The model under review builds one solid part; all positions refer to its coordinate system, in mm. Face numbers are marked on the shaded views. A direction names the side the tool comes from. Coordinates: 2 decimals unless noted, no trailing zeros. Write each loop counter-clockwise with the first axis right and the second up, starting at its lowest first coordinate (ties: lowest second). Pieces come first, ordered by that corner, then holes. Notation, with made-up numbers: (-8, -38.75) -> (14, -38.75) arc R31 ccw to (14, -6.75) -> close; hole circle Ø7 at (16.25, 70). An arc over 180 degrees is marked (long way). Put each result on its own line as item: value. Start each with the question number.
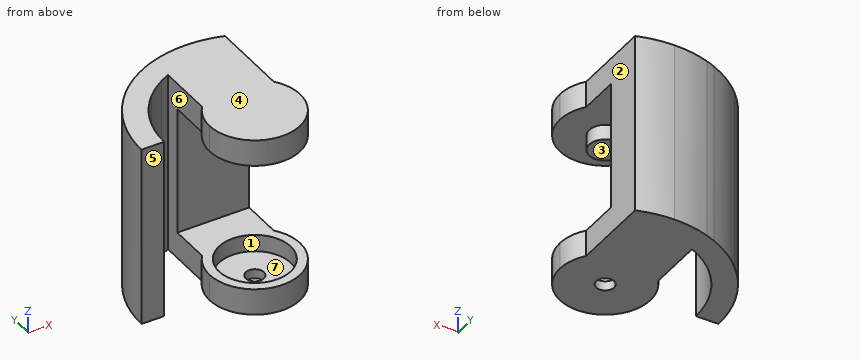
from build123d import *
from build123d.topology import SkipClean

# Parameters (mm, degrees)
SKETCH1_R           = 9.5
BOSS_EXTRUDE1_DEPTH = 48
SKETCH2_W           = 34
SKETCH2_H           = 30
CUT_EXTRUDE1_DEPTH  = 62.481704596
BOSS_EXTRUDE2_START = -2.5
SKETCH3_R           = 9.5
SKETCH3_R_2         = 2.4
BOSS_EXTRUDE2_DEPTH = 2.5
SKETCH4_R           = 9.5
SKETCH4_R_2         = 4.2
BOSS_EXTRUDE3_DEPTH = 7
SKETCH5_R           = 4.2
BOSS_EXTRUDE4_DEPTH = 11
CUT_EXTRUDE2_DEPTH  = 58.861904566
BOSS_EXTRUDE5_DEPTH = 48


with BuildPart() as part:
    # Sketch1 → Boss-Extrude1 (new body)
    with BuildSketch(Plane.XY):
        with BuildLine():
            Line((-12, 0), (-12, 30))
            Line((-12, 30), (12, 30))
            Line((12, 30), (12, 0))
            ThreePointArc((12, 0), (0, -12), (-12, 0))
        make_face()
        Circle(SKETCH1_R, mode=Mode.SUBTRACT)
    extrude(amount=-BOSS_EXTRUDE1_DEPTH)

    # Sketch2 → Cut-Extrude1 (cut, through all)
    with BuildSketch(Plane.ZY.offset(12)):
        with Locations((-24, 3)):
            Rectangle(SKETCH2_W, SKETCH2_H)
    extrude(amount=-CUT_EXTRUDE1_DEPTH, mode=Mode.SUBTRACT)

    # Sketch3 → Boss-Extrude2 (add)
    with BuildSketch(Plane(origin=(0, 0, -48), x_dir=(-1, 0, 0), z_dir=(0, 0, -1)).offset(BOSS_EXTRUDE2_START)):
        Circle(SKETCH3_R)
        Circle(SKETCH3_R_2, mode=Mode.SUBTRACT)
    extrude(amount=BOSS_EXTRUDE2_DEPTH)

    # Sketch4 → Boss-Extrude3 (add)
    with BuildSketch(Plane.XY):
        with Locations(Location((0, 0, 0), (0, 0, 180))):
            Circle(SKETCH4_R)
        Circle(SKETCH4_R_2, mode=Mode.SUBTRACT)
    extrude(amount=-BOSS_EXTRUDE3_DEPTH)

    # Sketch5 → Boss-Extrude4 (add)
    with BuildSketch(Plane.XY):
        Circle(SKETCH5_R)
    extrude(amount=-BOSS_EXTRUDE4_DEPTH)

    # Sketch6 → Cut-Extrude2 (cut, through all)
    with SkipClean():  # the faces are left unmerged after this step: merging them gives an invalid solid
        with BuildSketch(Plane(origin=(0, 0, -48), x_dir=(-1, 0, 0), z_dir=(0, 0, -1))):
            with BuildLine():
                Line((-12, 30), (-12, 27.49545417))
                ThreePointArc((-12, 27.49545417), (-10.760725498, 28.003692377), (-9.5, 28.45610655))
                Line((-9.5, 28.45610655), (-9.5, 30))
                Line((-9.5, 30), (-12, 30))
            make_face()
            with BuildLine():
                Line((-9.5, 30), (-9.5, 28.45610655))
                ThreePointArc((-9.5, 28.45610655), (-4.812317696, 29.611511248), (2.9e-08, 30))
                Line((2.9e-08, 30), (-9.5, 30))
            make_face()
            with BuildLine():
                ThreePointArc((2.9e-08, 30), (4.812317725, 29.611511243), (9.5, 28.45610655))
                Line((9.5, 28.45610655), (9.5, 30))
                Line((9.5, 30), (2.9e-08, 30))
            make_face()
            with BuildLine():
                Line((9.5, 30), (9.5, 28.45610655))
                ThreePointArc((9.5, 28.45610655), (10.760725498, 28.003692377), (12, 27.49545417))
                Line((12, 27.49545417), (12, 30))
                Line((12, 30), (9.5, 30))
            make_face()
            with BuildLine():
                Line((-12, 20.784609691), (-12, 0))
                ThreePointArc((-12, 0), (-11.357816692, 3.872983346), (-9.5, 7.331439149))
                Line((-9.5, 7.331439149), (-9.5, 22.039736841))
                ThreePointArc((-9.5, 22.039736841), (-10.768302375, 21.448628487), (-12, 20.784609691))
            make_face()
            with BuildLine():
                Line((-12, 27.49545417), (-12, 20.784609691))
                ThreePointArc((-12, 20.784609691), (-10.768302375, 21.448628487), (-9.5, 22.039736841))
                Line((-9.5, 22.039736841), (-9.5, 28.45610655))
                ThreePointArc((-9.5, 28.45610655), (-10.760725498, 28.003692377), (-12, 27.49545417))
            make_face()
            with BuildLine():
                Line((9.5, 22.039736841), (9.5, 9.5))
                Line((9.5, 9.5), (12, 12))
                Line((12, 12), (12, 20.784609691))
                ThreePointArc((12, 20.784609691), (10.768302375, 21.448628487), (9.5, 22.039736841))
            make_face()
            with BuildLine():
                ThreePointArc((9.5, 7.331439149), (11.357816692, 3.872983346), (12, 0))
                Line((12, 0), (12, 12))
                Line((12, 12), (9.5, 9.5))
                Line((9.5, 9.5), (9.5, 7.331439149))
            make_face()
        extrude(amount=-CUT_EXTRUDE2_DEPTH, mode=Mode.SUBTRACT)

    # Sketch7 → Boss-Extrude5 (add)
    with SkipClean():  # the faces are left unmerged after this step: merging them gives an invalid solid
        with BuildSketch(Plane(origin=(0, 0, -48), x_dir=(-1, 0, 0), z_dir=(0, 0, -1))):
            with BuildLine():
                ThreePointArc((12, 20.784609691), (14.610274296, 19.040480167), (16.970562748, 16.970562748))
                Line((16.970562748, 16.970562748), (21.213203436, 21.213203436))
                ThreePointArc((21.213203436, 21.213203436), (16.901061777, 24.786167732), (12, 27.49545417))
                Line((12, 27.49545417), (12, 20.784609691))
            make_face()
            with BuildLine():
                ThreePointArc((16.970562748, 16.970562748), (22.17310878, 9.184402377), (24, 0))
                Line((24, 0), (30, 0))
                ThreePointArc((30, 0), (27.716385975, 11.480502971), (21.213203436, 21.213203436))
                Line((21.213203436, 21.213203436), (16.970562748, 16.970562748))
            make_face()
        extrude(amount=-BOSS_EXTRUDE5_DEPTH)


solid = part.part
1. The part is to be moulded in two halves that separate along Y. For the marked faces 4, 5, 6 and 7, say which applies: released by +Y, released by -Y, zero draft, split by the parting line, or undercut.
2. Consider section B-B on z = -44.5. State the section outline as (x, y) points, then the cut area to 3 significant figures.
3. Wall thickness on line 1 (Y direction, x = 0, z = -44.25); line 2 (Z direction, x = -4.5, y = 15); line 3 (Y direction, x = 0, z = -46): over which ranges is each line inside the solid? List them lowest first. Write a range as from..to.
4. Tool access review of the marked faces 1, 2 and 3: name each direction out of +Z, -Z, +X, -X, +Y, -Y from which nothing blocks a thin tool from reaching the whole face with its end or side.
5. Consider section C-C on z = -15.5. State the section outline as (x, y) points, then the cut area to 3 significant figures.
6. Consider section D-D on x = -27. State the section outline as (y, z) points.
7. Insertion check: P1, Ø12, axis at y = 17.5, z = -14.5, coming from the -X side; P2, Ø10, axis at y = 12, z = -38.5, coming from the +X side; P3, Ø9.5, axis at x = -1.5, z = -16, coming from the -Y side; P4, Ø1, axis at x = -12.5, y = 5.5, coming from the +Z side. Each pin has a flat end and moves straight along its axis. Give the tip position at first contact, or say it passes through.
8. Consider section A-A on y = 1. State the section outline as (x, z) points, then the cut area to 3 significant figures.
Output values:
1. face 4: zero draft
1. face 5: released by -Y
1. face 6: undercut
1. face 7: undercut
2. outline: (-30, 0) -> (-24, 0) arc R24 cw to (-9.5, 22.04) -> (-9.5, 7.33) arc R12 ccw (long way) to (9.5, 7.33) -> (9.5, 28.46) arc R30 ccw to start; hole circle Ø19 at (0, 0)
2. area: 724 mm^2
3. line 1: y = -12..-9.5, 9.5..30
3. line 2: z = -48..-41, -7..0
3. line 3: y = -12..-2.4, 2.4..30
4. face 1: none
4. face 2: +Z, -Z, +X, +Y
4. face 3: +X, -Y
5. outline: (-30, 0) -> (-24, 0) arc R24 cw to (-9.5, 22.04) -> (-9.5, 18) -> (9.5, 18) -> (9.5, 28.46) arc R30 ccw to start
5. area: 415 mm^2
6. outline: (0, -48) -> (13.08, -48) -> (13.08, 0) -> (0, 0) -> close
7. P1: stops at x = -27.71
7. P2: stops at x = 9.5
7. P3: stops at y = 18
7. P4: passes through
8. outline: (-29.98, -48) -> (-23.98, -48) -> (-23.98, 0) -> (-29.98, 0) -> close; (-11.96, -48) -> (-2.18, -48) -> (-2.18, -45.5) -> (-9.45, -45.5) -> (-9.45, -41) -> (-11.96, -41) -> close; (-11.96, -7) -> (-4.08, -7) -> (-4.08, -11) -> (4.08, -11) -> (4.08, -7) -> (11.96, -7) -> (11.96, 0) -> (-11.96, 0) -> close; (2.18, -48) -> (11.96, -48) -> (11.96, -41) -> (9.45, -41) -> (9.45, -45.5) -> (2.18, -45.5) -> close
8. area: 560 mm^2
